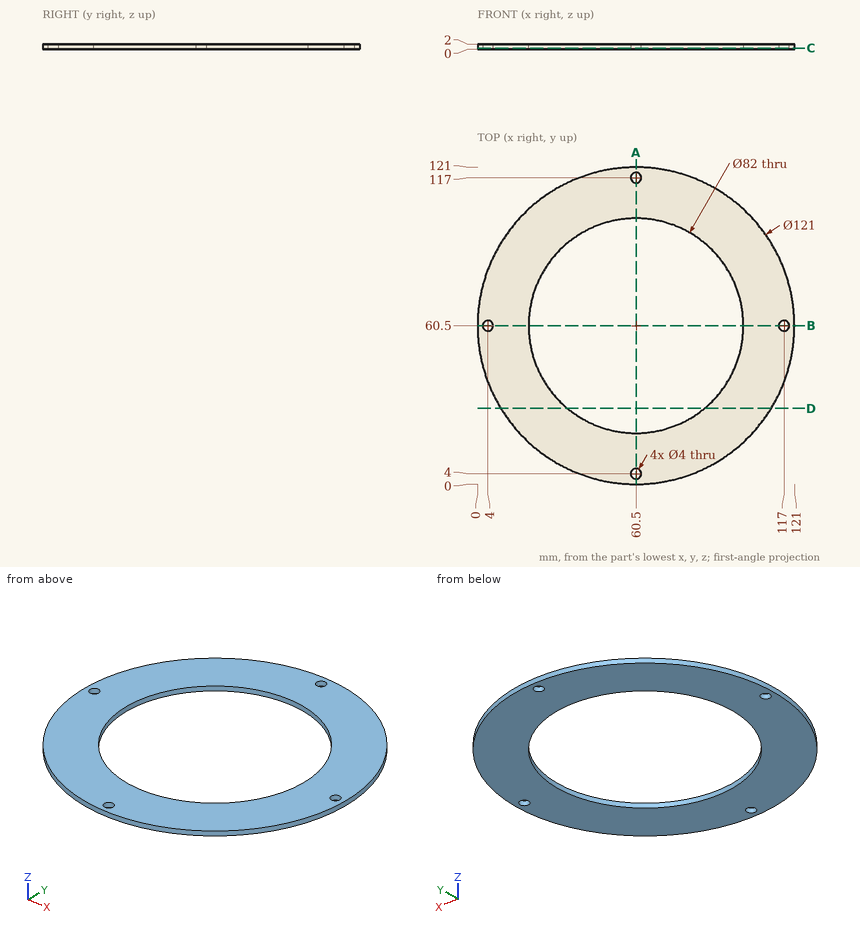
The figure shows three views and two pictorial views of one solid part (mm, origin at its lowest corner). Answer the questions. Coordinates: 2 decimals unless noted, no trailing zeros. Loops run counter-clockwise (first coordinate to the right, second up) from the corner with the lowest first, then second, coordinate; pieces in that order, holes last. Notation, with made-up numbers: (39.25, 60.25) - (63.25, 60.25) arc R21 ccw to (63.25, 75.25) - close; hole circle Ø9 at (-30.75, 61.25). An arc over 180 degrees is marked (long way). Use a Markdown table: item, result. Add a question column.
1) The part is cut by section D-D, the plane y = 29. Give the vertices of the cut face in (x, z).
2) The part is cut by section C-C, the plane z = 0.4. Give the vertices of the cut face in (x, y), and give its area (3 significant figures).
3) The part is cut by section A-A, the plane x = 60.5. Give the vertices of the cut face in (y, z).
4) Given pin 1 (3.5 mm diameter, centred on x = 60.5, y = 4, fed in from +Z), flat-ended and moving along its own axis, determine where the tip first touches the part or whether it passes through.
5) Find the intervals of material crossed by line 1 (Y direction, x = 60.5, z = 0.6); line 2 (Y direction, x = 83, z = 0.85); line 3 (Y direction, x = 47, z = 0.45), in increasing order.
Here are the results:
| question | item | result |
|---|---|---|
| 1 | outline | (8.85, 0) - (34.26, 0) - (34.26, 2) - (8.85, 2) - close; (86.74, 0) - (112.15, 0) - (112.15, 2) - (86.74, 2) - close |
| 2 | outline | circle Ø121 at (60.5, 60.5); hole circle Ø4 at (4, 60.5); hole circle Ø82 at (60.5, 60.5); hole circle Ø4 at (60.5, 4); hole circle Ø4 at (60.5, 117); hole circle Ø4 at (117, 60.5) |
| 2 | area | 6,170 mm^2 |
| 3 | outline | (0, 0) - (2, 0) - (2, 2) - (0, 2) - close; (6, 0) - (19.5, 0) - (19.5, 2) - (6, 2) - close; (101.5, 0) - (115, 0) - (115, 2) - (101.5, 2) - close; (119, 0) - (121, 0) - (121, 2) - (119, 2) - close |
| 4 | pin 1 | passes through |
| 5 | line 1 | y = 0 to 2, 6 to 19.5, 101.5 to 115, 119 to 121 |
| 5 | line 2 | y = 4.34 to 26.23, 94.77 to 116.66 |
| 5 | line 3 | y = 1.53 to 21.79, 99.21 to 119.47 |
